CAD build for the part. Positions are in the model's coordinates, mm. A direction names the side the tool comes from. Give positions to 0.01 mm unless a question says otherwise; leave off trailing zeros. Loops run counter-clockwise (first coordinate to the right, second up) from the corner with the lowest first, then second, coordinate; pieces in that order, holes last.
```python
from build123d import *

# Parameters (mm, degrees)
BOSS_EXTRUDE1_DEPTH = 14
SKETCH2_R           = 2.25
BOSS_EXTRUDE2_DEPTH = 2.75
SKETCH4_R           = 2.25
CUT_EXTRUDE1_DEPTH  = 2.75


with BuildPart() as part:
    # Sketch1 → Boss-Extrude1 (new body)
    with BuildSketch(Plane(origin=(0, 0, 0), x_dir=(1, 0, 0), z_dir=(0, 1, 0))):
        Polygon((8.692930554, 39.050653624), (32.692930554, 39.050653624), (32.692930554, 25.995392605), (35.192930554, 25.995392605), (35.192930554, 12.875501581), (25.138333129, -0.949346376), (15.571219536, -0.949346376), (6.192930554, 12.875501581), (6.192930554, 25.995392605), (8.692930554, 25.995392605), align=None)
    extrude(amount=BOSS_EXTRUDE1_DEPTH)

    # Sketch2 → Boss-Extrude2 (add)
    with BuildSketch(Plane.XZ):
        with Locations(Location((20.5, -18, 0), (0, 0, 270))):
            Circle(SKETCH2_R)
    extrude(amount=BOSS_EXTRUDE2_DEPTH)

    # Sketch4 → Cut-Extrude1 (cut)
    with BuildSketch(Plane(origin=(0, 0, 0), x_dir=(-1, 0, 0), z_dir=(0, -1, 0))):
        Polygon((-8.692930554, 30.050653624), (-8.692930554, 25.995392605), (-6.192930554, 25.995392605), (-6.192930554, 12.875501581), (-15.571219536, -0.949346376), (-25.138333129, -0.949346376), (-35.192930554, 12.875501581), (-35.192930554, 25.995392605), (-32.692930554, 25.995392605), (-32.692930554, 30.050653624), align=None)
        with Locations(Location((-20.5, 18, 0), (0, 0, 90))):
            Circle(SKETCH4_R, mode=Mode.SUBTRACT)
    extrude(amount=-CUT_EXTRUDE1_DEPTH, mode=Mode.SUBTRACT)


solid = part.part
```
1. Saw through at C-C, the plane z = -18. List the corners of the cut face in (x, y), and give its area (3 significant figures).
Responses:
outline: (6.19, 2.75) - (18.25, 2.75) - (18.25, -2.75) - (22.75, -2.75) - (22.75, 2.75) - (35.19, 2.75) - (35.19, 14) - (6.19, 14) - close
area: 351 mm2
2. Probe line 1 along Y through (x, z) = (8.25, -22); line 2 along X through (y, z) = (3.75, -36.5); line 3 along Z through (x, y) = (16, 2.5). List the from-to ranges inside material, lowest first.
Responses:
line 1: y = 2.75 to 14
line 2: x = 8.69 to 32.69
line 3: z = -39.05 to -30.05
3. Tool access for faces 1 (the face through (21, -2.75, -18)), 2 (the face through (34, 8, -25.995)), 3 (the face through (7, 8, -25.995)), 4 (the face through (21, 14, -19)), 5 (the face through (18.504, -0.038, -19.038)): list every direction of +Z, -Z, +X, -X, +Y, -Y with a clear straight run to the whole face (end or side of a thin tool).
Responses:
face 1: +Z, -Z, +X, -X, -Y
face 2: -Z, +X, +Y, -Y
face 3: -Z, -X, +Y, -Y
face 4: +Z, -Z, +X, -X, +Y
face 5: -Y
4. Drop flat-ended pins along their axis: pin 1 (10 mm diameter, centred on x = 20.5, z = -32.5, fed in from -Y); pin 2 (1 mm diameter, centred on x = 12.5, y = 6.5, fed in from +Z); pin 3 (4 mm diameter, centred on y = 4, z = -3, fed in from -X). Give the stop position or say it passes through.
Responses:
pin 1: stops at y = 0
pin 2: stops at z = -2.84
pin 3: stops at x = 11.54
5. Saw through at D-D, the plane x = 10.25. List the corners of the cut face in (y, z).
Responses:
outline: (0, -39.05) - (14, -39.05) - (14, -6.89) - (2.75, -6.89) - (2.75, -30.05) - (0, -30.05) - close
6. Saw through at B-B, the plane y = 6.5. List the corners of the cut face in (x, z), and give its area (3 significant figures).
Responses:
outline: (6.19, -26) - (8.69, -26) - (8.69, -39.05) - (32.69, -39.05) - (32.69, -26) - (35.19, -26) - (35.19, -12.88) - (25.14, 0.95) - (15.57, 0.95) - (6.19, -12.88) - close
area: 960 mm2
7. Saw through at A-A, the plane x = 20.5. List the corners of the cut face in (y, z), and give its area (4 significant figures).
Responses:
outline: (-2.75, -20.25) - (2.75, -20.25) - (2.75, -30.05) - (0, -30.05) - (0, -39.05) - (14, -39.05) - (14, 0.95) - (2.75, 0.95) - (2.75, -15.75) - (-2.75, -15.75) - close
area: 499.5 mm2
